Study the drawing (mm; zero at the part's minimum x, y, z) and answer. Coordinates: 2 decimals unless noted, no trailing zeros. Loops run counter-clockwise (first coordinate to the right, second up) from the corner with the lowest first, then second, coordinate; pieces in that order, holes last. Notation, with made-up numbers: (-36, -26.75) -> (16, -26.75) arc R12 cw to (16, -20.75) -> close; hole circle Ø7 at (-6.75, 25.5). An arc over 180 degrees is marked (long way). Answer as CSV lines item,"result".
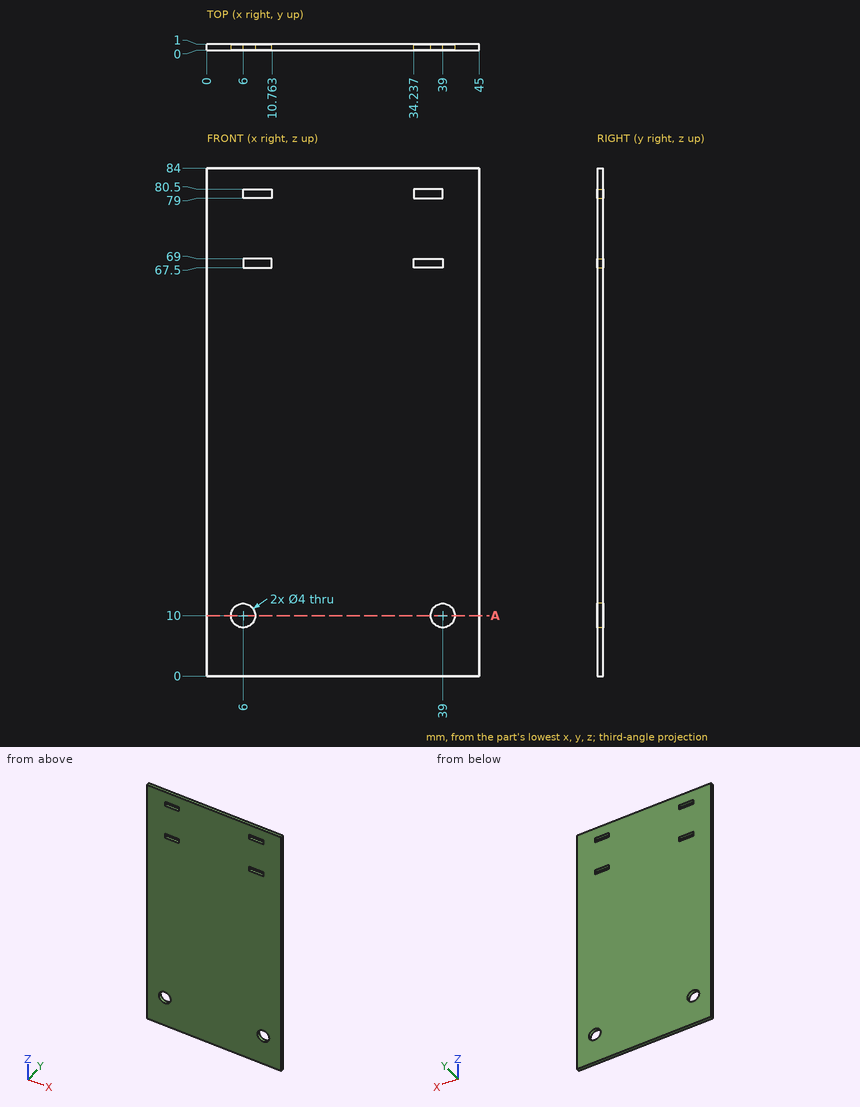
Q1. A cutting plane is placed at A-A, the plane z = 10. Write down the section's boundary in (x, y).
Results:
outline,"(0, 0) -> (4, 0) -> (4, 1) -> (0, 1) -> close; (8, 0) -> (37, 0) -> (37, 1) -> (8, 1) -> close; (41, 0) -> (45, 0) -> (45, 1) -> (41, 1) -> close"
Q2. Given pin 1 Ø2.5 at (x, z) = (6, 10) entering from -Y, flat-ended and moving along its own axis, determine where the tip first touches the part or whether it passes through.
Results:
pin 1,"passes through"
Q3. Find the intervals of material crossed by probe 1 along Z at (x, y) = (10, 0.9); probe 2 along Z at (x, y) = (6.5, 0.7) (1 decimal); probe 3 along Z at (x, y) = (40.5, 0.3) (1 decimal), in increasing order. Write a range as [from, to].
Results:
probe 1,"z = [0, 67.5], [69, 79], [80.5, 84]"
probe 2,"z = [0, 8.1], [11.9, 67.5], [69, 79], [80.5, 84]"
probe 3,"z = [0, 8.7], [11.3, 84]"
